Read the model definition and answer for the solid it produces. Units are mm, in the model's axes. A direction names the side the tool comes from. Coordinates: 2 decimals unless noted, no trailing zeros. Loops run counter-clockwise (first coordinate to the right, second up) from the corner with the lowest first, then second, coordinate; pieces in that order, holes last. Notation, with made-up numbers: (75, 45.5) - (117, 45.5) arc R19 cw to (117, 78.5) - close; hole circle Ø9 at (-23, 18.25). An arc over 180 degrees is marked (long way). One line per item, written item: value. Start each with the question number.
Autodesk Fusion 360 part; units mm, degrees
sketch "Sketch1" plane through (0, 0, 0) normal (0, 0, 1) x (1, 0, 0)
  line L0 (0, 0) -> (0, 70.4213)
  line L1 (0, 0) -> (8, 0)
  line L2 (8, 0) -> (8, 7)
  line L3 (8, 7) -> (6, 7)
  line L4 (6, 7) -> (6, 13)
  line L5 (6, 13) -> (8, 13)
  line L6 (8, 13) -> (8, 17)
  line L7 (8, 17) -> (0, 17)
  line L8 (2, 18.5) -> (2, 0)
  line L9 (5, 17) -> (5, 18.5)
  line L10 (5, 18.5) -> (0, 18.5)
  dimension "d1" = 17
  dimension "d2" = 4
  dimension "d3" = 7
  dimension "d4" = 12
  dimension "d5" = 16
  dimension "d6" = 1.5
  dimension "d7" = 10
  dimension "d8" = 4
revolve "Revolve1" add sketch "Sketch1" angle 360 about axis through (0, 0, 0) along (0, 1, 0) contours L1 L2 L3 L4 L5 L6 L7 L8 | L7 L8 L9 L10
sketch "Sketch2" plane through (0, 0, 0) normal (0, 1, 0) x (1, 0, 0)
  line L0 (0, 0) -> (6, 0) construction
  line L1 (0, 0) -> (-6, 0) construction
  circle A0 centre (-6, 0) radius 1
  circle A1 centre (6, 0) radius 1
  dimension "d10" = 2
  dimension "d11" = 6
extrude "Extrude1" cut sketch "Sketch2" along normal blind 5
chamfer "Chamfer1" distance 0.2 angle 45 4 edges at (-7.4586, 17, -2.8929) (-7.4586, 7, -2.8929) (-7.4586, 13, -2.8929) (-7.4586, 0, -2.8929)
1) Determine the mould class of faces 4 (the flat face through (4, 13, 5)), 5 (the cylindrical face through (5.2, 2.5, -0.6)), 6 (the flat face through (2, 17, 5)) for opening direction Y: released by +Y, released by -Y, zero draft, split by the parting line, or undercut.
2) Section C-C, the plane y = 3 is taken. Determine the outline of the cut face in (x, z), and give its area (3 significant figures).
3) Section A-A, the plane x = 0 is taken. Determine the outline of the cut face in (y, z).
4) Straight lines are drawn through the part: L1, parallel to X at y = 1.7, z = 0; L2, parallel to Y at x = 4.25, z = 5; L3, parallel to X at y = 9, z = 0. For each, find the intervals that lie inside material, in ascending order.
5) Flat-ended cylindrical pins translate along their axes: P1, Ø1, axis at y = 16, z = 6, coming from the +X side; P2, Ø1, axis at y = 13, z = 5.5, coming from the -X side; P3, Ø1.5, axis at y = 10.5, z = -1, coming from the +X side. Find the tip coordinate at first contact, or state that the pin passes through.
6) Section B-B, the plane y = 17.5 is taken. Determine the outline of the cut face in (x, z).
7) Section D-D, the plane y = 14.5 is taken. Determine the outline of the cut face in (x, z).
8) For faces 1 (the cylindrical face through (-1.08, 17.76, 4.88)), 2 (the cylindrical face through (-6.8, 2.5, -0.6)), 3 (the flat face through (4, 7, 5)), determine the directions among +Z, -Z, +X, -X, +Y, -Y from which every point of the face is accessible in a straight line to the end or side of a thin tool.
Answer below:
1. face 4: undercut
1. face 5: zero draft
1. face 6: released by +Y
2. outline: circle Ø16 at (0, 0); hole circle Ø2 at (-6, 0); hole circle Ø4 at (0, 0); hole circle Ø2 at (6, 0)
2. area: 182 mm2
3. outline: (0, -7.8) - (0.2, -8) - (6.8, -8) - (7, -7.8) - (7, -6) - (13, -6) - (13, -7.8) - (13.2, -8) - (16.8, -8) - (17, -7.8) - (17, -5) - (18.5, -5) - (18.5, -2) - (0, -2) - close; (0, 2) - (18.5, 2) - (18.5, 5) - (17, 5) - (17, 7.8) - (16.8, 8) - (13.2, 8) - (13, 7.8) - (13, 6) - (7, 6) - (7, 7.8) - (6.8, 8) - (0.2, 8) - (0, 7.8) - close
4. L1: -8 to -7, -5 to -2, 2 to 5, 7 to 8
4. L2: 0 to 7, 13 to 17
4. L3: -6 to -2, 2 to 6
5. P1: x = 5.81
5. P2: x = -6.21
5. P3: x = 5.99
6. outline: circle Ø10 at (0, 0); hole circle Ø4 at (0, 0)
7. outline: circle Ø16 at (0, 0); hole circle Ø4 at (0, 0)
8. face 1: +Y
8. face 2: -Y
8. face 3: none
